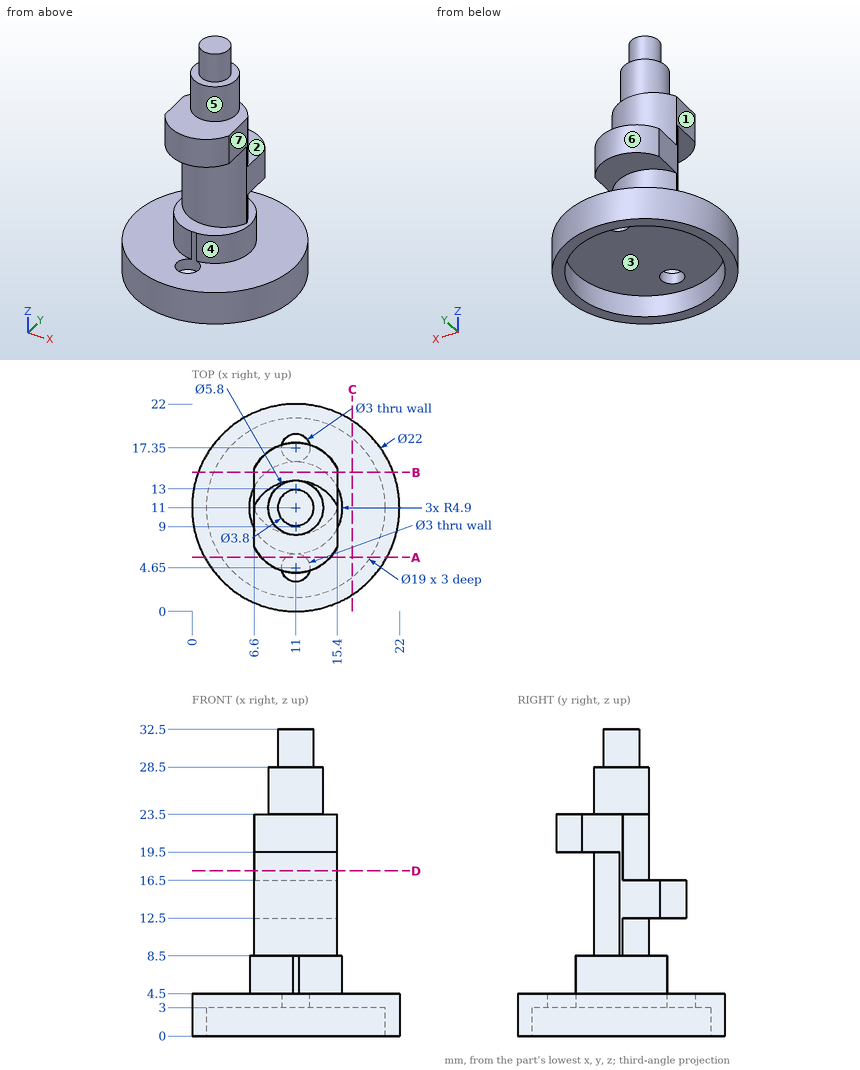
The figure shows three views and two pictorial views of one solid part (mm, origin at its lowest corner). Answer the questions. A direction names the side the tool comes from. Coordinates: 2 decimals unless noted, no trailing zeros. Order: outer loops, then holes, each group sorted by start corner. A loop starts at its lowest first (then second) coordinate and runs counter-clockwise, first axis right, second up. Notation, with made-up numbers: M -30.75,77.25 L 1.25,77.25 A14 ccw 1.25,102.25 Z; hole C -36,-24 d5. An arc over 180 degrees is marked long. Use CSV: the item, a comma, the result in double quotes.
1) Section B-B on y = 14.75 is taken. Write down the section's boundary in (x, z).
Worked out:
outline,"M 0.66,0 L 2.27,0 L 2.27,3 L 19.73,3 L 19.73,0 L 21.34,0 L 21.34,4.5 L 14.15,4.5 L 14.15,8.5 L 7.85,8.5 L 7.85,4.5 L 0.66,4.5 Z; M 6.6,12.5 L 15.4,12.5 L 15.4,16.5 L 6.6,16.5 Z"
2) For the marked faces 5, 6 and 7, determine the directions among +Z, -Z, +X, -X, +Y, -Y from which every point of the face is accessible in a straight line to the end or side of a thin tool.
Worked out:
face 5,"+Z"
face 6,"+Z, +Y"
face 7,"+Z, +X, +Y, -Y"
3) Determine the mould class of the marked faces 1, 2, 3 and 4 for opening direction Z: released by +Z, released by -Z, zero draft, split by the parting line, or undercut.
Worked out:
face 1,"zero draft"
face 2,"released by +Z"
face 3,"released by -Z"
face 4,"undercut"
4) Section C-C on x = 17 is taken. Write down the section's boundary in (y, z).
Worked out:
outline,"M 1.78,0 L 3.63,0 L 3.63,3 L 18.37,3 L 18.37,0 L 20.22,0 L 20.22,4.5 L 1.78,4.5 Z"
5) Section A-A on y = 5.75 is taken. Write down the section's boundary in (x, z).
Worked out:
outline,"M 1.33,0 L 3.08,0 L 3.08,3 L 9.98,3 L 9.98,4.5 L 1.33,4.5 Z; M 7.33,19.5 L 14.67,19.5 L 14.67,23.5 L 7.33,23.5 Z; M 12.02,3 L 18.92,3 L 18.92,0 L 20.67,0 L 20.67,4.5 L 12.02,4.5 Z"
6) Consider line 1 (Z direction, x = 7.75, y = 7.5); line 2 (Y direction, x = 11, z = 1.15); line 3 (Z direction, x = 10.5, y = 17.75). Determine where each line is inside the solid, lowest interval first. Write a range as [from, to].
Worked out:
line 1,"z = [3, 8.5], [19.5, 23.5]"
line 2,"y = [0, 1.5], [20.5, 22]"
line 3,"z = [12.5, 16.5]"
7) Flat-ended cylindrical pins translate along their axes: pin 1 Ø9 at (y, z) = (9.5, 16.5) entering from -X; pin 2 Ø2 at (x, y) = (11, 14) entering from -Z; pin 3 Ø5 at (y, z) = (13.5, 5.5) entering from +X. Find the tip coordinate at first contact, or state that the pin passes through.
Worked out:
pin 1,"stops at x = 6.6"
pin 2,"stops at z = 3"
pin 3,"stops at x = 22"
8) Section D-D on z = 17.5 is taken. Write down the section's boundary in (x, y), plus the area to 3 significant figures.
Worked out:
outline,"M 6.6,10.84 A4.9 ccw 15.4,10.84 L 15.4,11.16 A4.9 ccw 6.6,11.16 Z"
area,"37.3 mm^2"
